from build123d import *

# Parameters (mm, degrees)
SKETCH2_R           = 1.5
BOSS_EXTRUDE1_DEPTH = 30
BOSS_EXTRUDE2_DEPTH = 32
FILLET3_R           = 1
CUT_EXTRUDE1_DEPTH  = 13.5
SKETCH5_R           = 1.3
CUT_EXTRUDE2_DEPTH  = 10.517452338
SKETCH6_R           = 3
CUT_EXTRUDE3_DEPTH  = 28


with BuildPart() as part:
    # Sketch2 → Boss-Extrude1 (new body)
    with BuildSketch(Plane(origin=(0, 0, 0), x_dir=(1, 0, 0), z_dir=(0, 1, 0))):
        with BuildLine():
            Line((-12.939762178, 2.094266176), (-24.821781773, 3.29179515))
            ThreePointArc((-24.821781773, 3.29179515), (-30.987291256, -0.071668068), (-24.821747911, -3.435069212))
            Line((-24.821747911, -3.435069212), (-12.987160246, -2.166440487))
            ThreePointArc((-12.987160246, -2.166440487), (-10.8566751, -0.059524017), (-12.939762178, 2.094266176))
        make_face()
        with Locations((-26.987114413, 0)):
            Circle(SKETCH2_R, mode=Mode.SUBTRACT)
    extrude(amount=BOSS_EXTRUDE1_DEPTH)

    # Sketch2_3 → Boss-Extrude2 (add)
    with BuildSketch(Plane(origin=(0, 0, 0), x_dir=(1, 0, 0), z_dir=(0, 1, 0))):
        with BuildLine():
            Line((-26.987114411, -4.57148105), (-25.802758185, -4.412822706))
            ThreePointArc((-25.802758185, -4.412822706), (-24.779096258, -3.992509307), (-23.88896632, -3.335078105))
            Line((-23.88896632, -3.335078105), (-24.821747911, -3.435069212))
            ThreePointArc((-24.821747911, -3.435069212), (-30.987291256, -0.071668068), (-24.821781773, 3.29179515))
            Line((-24.821781773, 3.29179515), (-23.896053235, 3.198495628))
            ThreePointArc((-23.896053235, 3.198495628), (-24.802641315, 3.862379952), (-25.845447528, 4.2809484))
            Line((-25.845447528, 4.2809484), (-26.987114411, 4.428185187))
            ThreePointArc((-26.987114411, 4.428185187), (-31.48694753, -0.071647931), (-26.987114411, -4.57148105))
        make_face()
        with BuildLine():
            Line((-25.802758185, -4.412822706), (-12.637077878, -2.649126119))
            ThreePointArc((-12.637077878, -2.649126119), (-13.508046926, -2.620506326), (-14.322115833, -2.309543319))
            Line((-14.322115833, -2.309543319), (-23.88896632, -3.335078105))
            ThreePointArc((-23.88896632, -3.335078105), (-24.779096258, -3.992509307), (-25.802758185, -4.412822706))
        make_face()
        with BuildLine():
            ThreePointArc((-14.328363864, 2.234216353), (-13.517942982, 2.546845227), (-12.649914094, 2.579166576))
            Line((-12.649914094, 2.579166576), (-25.845447528, 4.2809484))
            ThreePointArc((-25.845447528, 4.2809484), (-24.802641315, 3.862379952), (-23.896053235, 3.198495628))
            Line((-23.896053235, 3.198495628), (-14.328363864, 2.234216353))
        make_face()
        with BuildLine():
            ThreePointArc((-12.637077878, -2.649126119), (-11.057896416, -1.833001646), (-10.355629468, -0.2))
            Line((-10.355629468, -0.2), (-10.371987074, 0.3))
            ThreePointArc((-10.371987074, 0.3), (-11.122262116, 1.828060363), (-12.649914094, 2.579166576))
            ThreePointArc((-12.649914094, 2.579166576), (-13.517942982, 2.546845227), (-14.328363864, 2.234216353))
            Line((-14.328363864, 2.234216353), (-12.939762178, 2.094266176))
            ThreePointArc((-12.939762178, 2.094266176), (-11.463920967, 1.453898193), (-10.856543276, -0.035823517))
            ThreePointArc((-10.856543276, -0.035823517), (-11.480586539, -1.542397225), (-12.987160246, -2.166440487))
            Line((-12.987160246, -2.166440487), (-14.322115833, -2.309543319))
            ThreePointArc((-14.322115833, -2.309543319), (-13.508046926, -2.620506326), (-12.637077878, -2.649126119))
        make_face()
        with BuildLine():
            ThreePointArc((-12.649914094, 2.579166576), (-11.122262116, 1.828060363), (-10.371987074, 0.3))
            Line((-10.371987074, 0.3), (-5.980159731, 0.3))
            Line((-5.980159731, 0.3), (-5.980159731, 1.71899167))
            Line((-5.980159731, 1.71899167), (-12.649914094, 2.579166576))
        make_face()
        with BuildLine():
            Line((-5.980021524, -1.757335699), (-5.980297938, -0.2))
            Line((-5.980297938, -0.2), (-10.355629468, -0.2))
            ThreePointArc((-10.355629468, -0.2), (-11.057896416, -1.833001646), (-12.637077878, -2.649126119))
            Line((-12.637077878, -2.649126119), (-5.980021524, -1.757335699))
        make_face()
    extrude(amount=BOSS_EXTRUDE2_DEPTH)

    # Fillet3
    fillet3_edges = [part.edges().sort_by_distance(p)[0] for p in [
        (-5.980159731, 16, -0.3),
        (-5.980297938, 16, 0.2),
    ]]
    fillet(fillet3_edges, radius=FILLET3_R)

    # Sketch4 → Cut-Extrude1 (cut)
    with BuildSketch(Plane(origin=(-10.351093889, 0, 0.338638235), x_dir=(-0.032697719, 0, -0.999465287), z_dir=(0.999465287, 0, -0.032697719))):
        Polygon((0.634009108, 16), (0.638979906, 2), (0.190205723, 2), (0.138712406, 16), align=None)
        Polygon((0.190205723, 30), (0.138712406, 16), (0.634009108, 16), (0.638979906, 30), align=None)
    extrude(amount=-CUT_EXTRUDE1_DEPTH, mode=Mode.SUBTRACT)

    # Sketch5 → Cut-Extrude2 (cut, through all)
    with BuildSketch(Plane(origin=(0.125841463, 0, 0.939384066), x_dir=(0.991146125, 0, -0.132775595), z_dir=(0.132775595, 0, 0.991146125))):
        with Locations((-8.160406455, 28)):
            Circle(SKETCH5_R)
        with Locations((-8.160406455, 4)):
            Circle(SKETCH5_R)
    extrude(amount=-CUT_EXTRUDE2_DEPTH, mode=Mode.SUBTRACT)

    # Sketch6 → Cut-Extrude3 (cut)
    with BuildSketch(Plane.XZ):
        with Locations((-26.987114413, 0)):
            Circle(SKETCH6_R)
    extrude(amount=-CUT_EXTRUDE3_DEPTH, mode=Mode.SUBTRACT)


solid = part.part
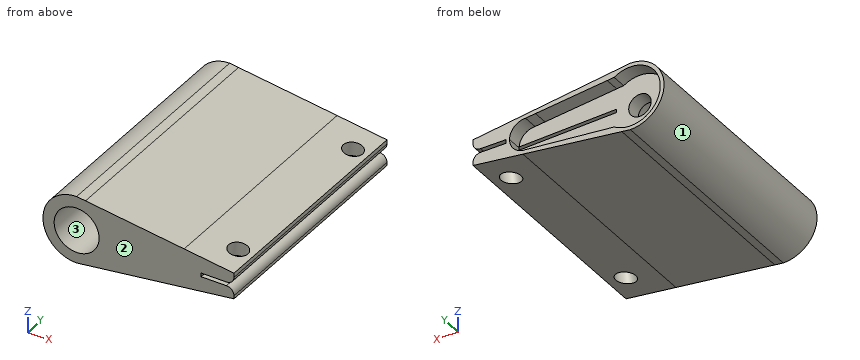
The listing builds one solid part. Answer for the finished solid, in the listing's coordinates (mm). Face numbers are marked on the shaded views. Coordinates: 2 decimals unless noted, no trailing zeros. Loops run counter-clockwise (first coordinate to the right, second up) from the corner with the lowest first, then second, coordinate; pieces in that order, holes last. Notation, with made-up numbers: (68.25, 43.5) -> (82.25, 43.5) arc R28 ccw to (82.25, 61.5) -> close; hole circle Ø7 at (85, 47). An arc over 180 degrees is marked (long way). Write item = value, one per line. Start each with the question number.
1) The mould has two halves that part along Z. Classify the marked faces 1, 2 and 3: released by +Z, released by -Z, zero draft, split by the parting line, or undercut.
2) A cutting plane is placed at B-B (x = -27.75). Give the vertices of the cut face in (y, z), then the cut area to 3 significant figures.
3) A cutting plane is placed at C-C (x = -18.5). Give the vertices of the cut face in (y, z), then the cut area to 3 significant figures.
4) Straight lines are drawn through the part: line 1 (X direction, y = 3, z = 0.75); line 2 (Y direction, x = -28, z = 2); line 3 (X direction, y = 26, z = -1.5). For each, find the intervals that lie inside material, in ascending order. Write a range as from..to.
5) Given pin 1 Ø10 at (x, y) = (-15, 21) entering from +Z; pin 2 Ø2.5 at (x, y) = (-9.5, 16) entering from +Z; pin 3 Ø5 at (x, y) = (-18, 12) entering from -Z, each flat-ended and moving along its own axis, determine where each tip first touches the part or whether it passes through.
Responses:
q1.face_1 = split by the parting line
q1.face_2 = zero draft
q1.face_3 = undercut
q2.outline = (0, -4.36) -> (32, -4.36) -> (32, -3.86) -> (30, -3.86) -> (30, -1.29) -> (28, -1.29) -> (28, -2.9) -> (0, -2.9) -> close; (0, 2.9) -> (28, 2.9) -> (28, 1.29) -> (30, 1.29) -> (30, 4) -> (32, 4) -> (32, 4.51) -> (0, 4.51) -> close
q2.area = 100 mm²
q3.outline = (0, -3.33) -> (32, -3.33) -> (32, -2.65) -> (30, -2.65) -> (30, -0.03) -> (16, -0.03) -> (2, -0.03) -> (2, 0.41) -> (16, 0.47) -> (30, 0.41) -> (30, 2.76) -> (32, 2.76) -> (32, 3.43) -> (0, 3.43) -> close
q3.area = 193 mm²
q4.line_1 = -31.44..-29.89, -24.08..-8.97, -7.29..-6.09
q4.line_2 = 28..30
q4.line_3 = -31.2..-29.59, -24.39..-5.98
q5.pin_1 = 3.64
q5.pin_2 = 2.4
q5.pin_3 = -3.59
